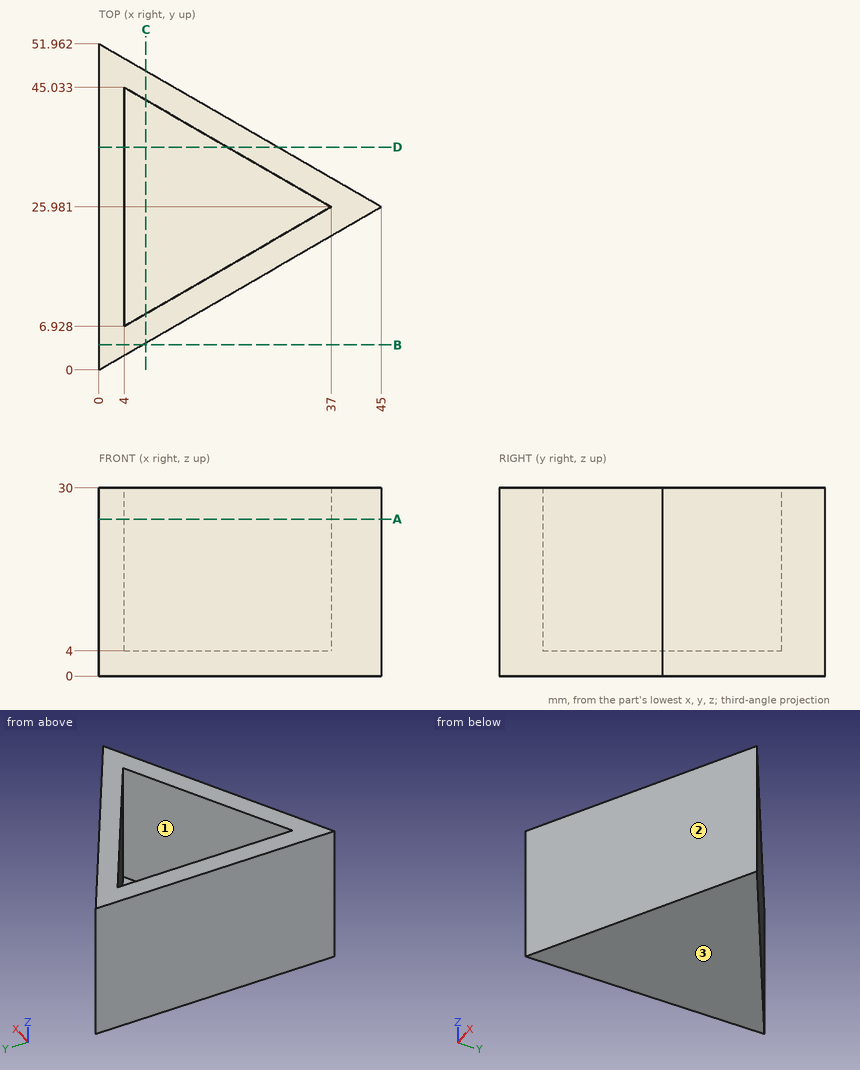
Can you work these out from the drawing? Everything is in mm from the part's minimum corner. Coordinates: 2 decimals unless noted, no trailing zeros. Loops run counter-clockwise (first coordinate to the right, second up) from the corner with the lowest first, then second, coordinate; pieces in that order, holes last.
1. Imagine slicing it at D-D, the plane y = 35.5. Please give me the cut outline in (x, z), and give its area (3 significant figures).
2. Imagine slicing it at B-B, the plane y = 4. Please give me the cut outline in (x, z).
3. For P1, Ø4, axis at x = 16, z = 8, coming from the +Y side; P2, Ø10, axis at x = 17.5, y = 29.5, coming from the +Z side; P3, Ø8, axis at x = 17, z = 16.5, coming from the +Y side (1 decimal), each with a flat end and sliding along its axis, tell me the tip position at first contact or that it passes through.
4. I need wall thicknesses on L1, parallel to Z at x = 6.5, y = 36.5; L2, parallel to X at y = 12, z = 12.25 (1 decimal); L3, parallel to X at y = 31.5, z = 15.25. Which ranges of each line are inside material? Lowest first, please.
5. Imagine slicing it at C-C, the plane x = 7.5. Please give me the cut outline in (y, z).
6. Imagine slicing it at A-A, the plane z = 25. Please give me the cut outline in (x, y).
7. If we mould it in two halves opening along Y, with no side actions, what happens to the marked faces 1, 2 and 3? For each: pulls with the +Y half, pulls with the -Y half, needs draft (parallel to the pull), parting line crosses it, or undercut.
Taken from the geometry:
1. outline: (0, 0) - (28.51, 0) - (28.51, 30) - (20.51, 30) - (20.51, 4) - (4, 4) - (4, 30) - (0, 30) - close
1. area: 426 mm2
2. outline: (0, 0) - (6.93, 0) - (6.93, 30) - (0, 30) - close
3. P1: stops at y = 43.88
3. P2: stops at z = 4
3. P3: stops at y = 44.5
4. L1: z = 0 to 4
4. L2: x = 0 to 4, 12.8 to 20.8
4. L3: x = 0 to 4, 27.44 to 35.44
5. outline: (4.33, 0) - (47.63, 0) - (47.63, 30) - (43.01, 30) - (43.01, 4) - (8.95, 4) - (8.95, 30) - (4.33, 30) - close
6. outline: (0, 0) - (45, 25.98) - (0, 51.96) - close; hole (4, 6.93) - (37, 25.98) - (4, 45.03) - close
7. face 1: undercut
7. face 2: pulls with the -Y half
7. face 3: needs draft
